```python
from build123d import *

# Parameters (mm, degrees)
SKETCH1_W           = 50.8
SKETCH1_H           = 44.45
BOSS_EXTRUDE1_DEPTH = 25.4
SKETCH4_R           = 2
CUT_EXTRUDE3_DEPTH  = 73.122135992
SKETCH5_W           = 50.8
SKETCH5_H           = 12.7
CUT_EXTRUDE4_DEPTH  = 6.35
SKETCH6_R           = 2.032
CUT_EXTRUDE5_DEPTH  = 71.138042459


with BuildPart() as part:
    # Sketch1 → Boss-Extrude1 (new body)
    with BuildSketch(Plane.XY):
        with Locations((25.4, 22.225)):
            Rectangle(SKETCH1_W, SKETCH1_H)
    extrude(amount=BOSS_EXTRUDE1_DEPTH)

    # Sketch4 → Cut-Extrude3 (cut, through all)
    with BuildSketch(Plane(origin=(0, 44.45, 0), x_dir=(1, 0, 0), z_dir=(0, 1, 0))):
        with Locations(Location((6.35, -12.7, 0), (0, 0, 270))):
            Circle(SKETCH4_R)
        with Locations(Location((44.45, -12.7, 0), (0, 0, 270))):
            Circle(SKETCH4_R)
    extrude(amount=-CUT_EXTRUDE3_DEPTH, mode=Mode.SUBTRACT)

    # Sketch5 → Cut-Extrude4 (cut)
    with BuildSketch(Plane.XY.offset(25.4)):
        with Locations((25.4, 22.225)):
            Rectangle(SKETCH5_W, SKETCH5_H)
    extrude(amount=-CUT_EXTRUDE4_DEPTH, mode=Mode.SUBTRACT)

    # Sketch6 → Cut-Extrude5 (cut, through all)
    with BuildSketch(Plane.XY.offset(19.05)):
        with Locations((25.4, 22.225)):
            Circle(SKETCH6_R)
        with Locations((38.1, 22.225)):
            Circle(SKETCH6_R)
        with Locations((12.7, 22.225)):
            Circle(SKETCH6_R)
    extrude(amount=-CUT_EXTRUDE5_DEPTH, mode=Mode.SUBTRACT)


solid = part.part
```
Source: CAD feature listing. Evaluate the final solid. Frame: model axes, mm. A direction names the side the tool comes from. Give positions to 0.01 mm unless a question says otherwise; leave off trailing zeros. Write each loop counter-clockwise with the first axis right and the second up, starting at its lowest first coordinate (ties: lowest second). Pieces come first, ordered by that corner, then holes. Notation, with made-up numbers: (-36.75, 51) - (15.25, 51) arc R16 ccw to (15.25, 63) - close; hole circle Ø7 at (7, 30.5). An arc over 180 degrees is marked (long way). One line per item, written item: value. Start each with the question number.
Q1. Section query A-A, the plane x = 12.7. Return the cut outline in (y, z) (3 decimals).
Q2. Section query D-D, the plane y = 26. Return the cut outline in (x, z), then the cut area to 3 significant figures.
Q3. Section query B-B, the plane z = 12.7. Return the cut outline in (x, y) (3 decimals).
Q4. Draft query along X for faces 1 (the face through (50.8, 22, 13)), 2 (the face through (36.07, 22.31, 9.66)), 3 (the face through (25, 28.575, 22)). Return one class per face: +X half, -X half, draft (parallel to the pull), parting line (faces both ways), or undercut.
Q5. Material intervals for probe 1 along X at (y, z) = (12.5, 11); probe 2 along X at (y, z) = (21.5, 7.5); probe 3 along Y at (x, z) = (12.7, 6.25), sorted ascending. Write a range as from..to.
Q6. Section query C-C, the plane x = 19.5. Return the cut outline in (y, z) (3 decimals).
Q7. First-contact query: pin 1 Ø5.5 at (x, y) = (25.4, 22.225) entering from +Z; pin 2 Ø3 at (x, z) = (6.35, 12.7) entering from +Y. Flat tips, straight axial feed; report the tip coordinate or a pass-through.
Q8. Set-up query: faces 4 (the face through (25, 15.875, 22)), 5 (the face through (27.28, 21.45, 9.66)). Return all of +Z, -Z, +X, -X, +Y, -Y with unobstructed straight access to the full face (end or side cutting, diameter ignored); none if empty.
Answer:
1. outline: (0, 0) - (20.193, 0) - (20.193, 19.05) - (15.875, 19.05) - (15.875, 25.4) - (0, 25.4) - close; (24.257, 0) - (44.45, 0) - (44.45, 25.4) - (28.575, 25.4) - (28.575, 19.05) - (24.257, 19.05) - close
2. outline: (0, 0) - (50.8, 0) - (50.8, 19.05) - (0, 19.05) - close; hole circle Ø4 at (6.35, 12.7); hole circle Ø4 at (44.45, 12.7)
2. area: 943 mm2
3. outline: (0, 0) - (4.35, 0) - (4.35, 44.45) - (0, 44.45) - close; (8.35, 0) - (42.45, 0) - (42.45, 44.45) - (8.35, 44.45) - close; (46.45, 0) - (50.8, 0) - (50.8, 44.45) - (46.45, 44.45) - close; hole circle Ø4.064 at (12.7, 22.225); hole circle Ø4.064 at (25.4, 22.225); hole circle Ø4.064 at (38.1, 22.225)
4. face 1: +X half
4. face 2: undercut
4. face 3: draft
5. probe 1: x = 0..5.3, 7.4..43.4, 45.5..50.8
5. probe 2: x = 0..10.8, 14.6..23.5, 27.3..36.2, 40..50.8
5. probe 3: y = 0..20.19, 24.26..44.45
6. outline: (0, 0) - (44.45, 0) - (44.45, 25.4) - (28.575, 25.4) - (28.575, 19.05) - (15.875, 19.05) - (15.875, 25.4) - (0, 25.4) - close
7. pin 1: stops at z = 19.05
7. pin 2: passes through
8. face 4: +Z, +X, -X
8. face 5: +Z, -Z
